Geometry check sheet. Reference: drawing and pictorial views, mm from the part's lowest x, y, z. A direction names the side the tool comes from. Coordinates: 2 decimals unless noted, no trailing zeros. Loops run counter-clockwise (first coordinate to the right, second up) from the corner with the lowest first, then second, coordinate; pieces in that order, holes last. Notation, with made-up numbers: (-25, 22) - (21, 22) arc R21 ccw to (21, 39) - close; hole circle Ø10 at (-35.75, -39). An arc over 180 degrees is marked (long way). Write each question's results on one line, items separated by ' | '. Start each with the question number.
1. Cross-section at A-A (z = 2.75). Give the number of separate pieces and of enclosed holes in the cut face, and give its area (3 significant figures).
2. Cross-section at C-C (y = 11). Record the cut outline in (x, z), and give its area (3 significant figures).
3. Draft check along X on the marked faces 1, 2 and 3. Enter one of: released by +X, released by -X, zero draft, split by the parting line, or undercut.
4. Tool access check on the marked faces 4, 5 and 6. Record the directions out of +Z, -Z, +X, -X, +Y, -Y that give a thin tool (end or side, any length) a straight path to the whole face; none if there is none.
5. Cross-section at B-B (x = 65). Record the cut outline in (y, z), and give its area (3 significant figures).
6. Thickness scan on line 1 (X direction, y = 19, z = 4); line 2 (Y direction, x = 65, z = 7); line 3 (X direction, y = 24.5, z = 4.5) (1 decimal). Record the ranges inside material, lowest first. Write a range as [from, to].
7. Cross-section at D-D (x = 11). Record the cut outline in (y, z).
8. Gauge pin test, flat ends, axial feed: P1, Ø7, axis at x = 10, y = 19, coming from the +Z side; P2, Ø5.5, axis at x = 74.53, y = 13.5, coming from the -Z side; P3, Ø4, axis at y = 6.5, z = 3, coming from the +X side (1 decimal); P4, Ø4.5, axis at x = 29, z = 5.5, coming from the +Y side. Record the tip position at first contact, or that the pin passes through.
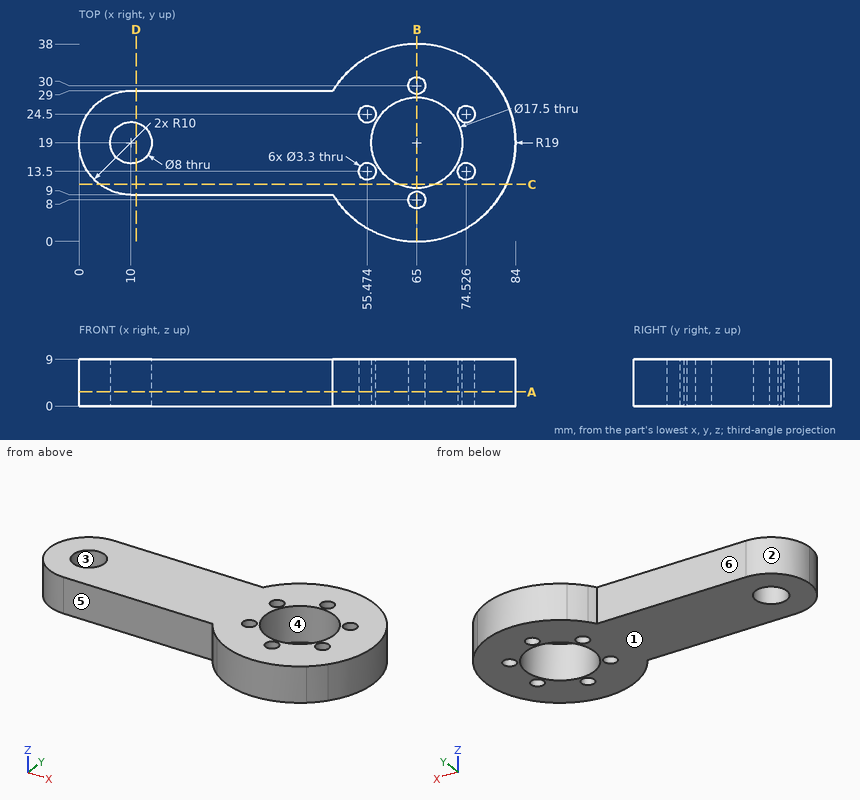
Established:
1) separate pieces: 1 | enclosed holes: 8 | area: 1,690 mm^2
2) outline: (4, 0) - (61.46, 0) - (61.46, 9) - (4, 9) - close; (68.54, 0) - (82.23, 0) - (82.23, 9) - (68.54, 9) - close | area: 640 mm^2
3) face 1: zero draft | face 2: released by -X | face 3: undercut
4) face 4: +Z, -Z | face 5: +Z, -Z, -X, -Y | face 6: +Z, -Z, -X, +Y
5) outline: (0, 0) - (6.35, 0) - (6.35, 9) - (0, 9) - close; (9.65, 0) - (10.25, 0) - (10.25, 9) - (9.65, 9) - close; (27.75, 0) - (28.35, 0) - (28.35, 9) - (27.75, 9) - close; (31.65, 0) - (38, 0) - (38, 9) - (31.65, 9) - close | area: 125 mm^2
6) line 1: [0, 6], [14, 56.25], [73.75, 84] | line 2: [0, 6.35], [9.65, 10.25], [27.75, 28.35], [31.65, 38] | line 3: [1.6, 53.8], [57.1, 58.2], [71.8, 72.9], [76.2, 83.2]
7) outline: (9, 0) - (15.13, 0) - (15.13, 9) - (9, 9) - close; (22.87, 0) - (29, 0) - (29, 9) - (22.87, 9) - close
8) P1: through | P2: z = 0 | P3: x = 80.8 | P4: y = 29
